```python
from build123d import *

# Parameters (mm, degrees)
SKETCH1_W             = 70
SKETCH1_H             = 5
BOSS_EXTRUDE1_DEPTH   = 36
SKETCH1_W_2           = 15
BOSS_EXTRUDE1_2_DEPTH = 36
SKETCH2_W             = 6
SKETCH2_H             = 70
BOSS_EXTRUDE2_DEPTH   = 70
M2_TAPPED_HOLE1_D     = 1.6
M2_TAPPED_HOLE1_DEPTH = 5
M2_TAPPED_HOLE1_TIP   = 0.480688495
M3_TAPPED_HOLE1_D     = 2.5
M2_5_TAPPED_HOLE1_D   = 2.05
SKETCH10_W            = 16.15
SKETCH10_H            = 7.752972879
CUT_EXTRUDE1_DEPTH    = 10


with BuildPart() as part:
    # Sketch1 → Boss-Extrude1 (new body)
    with BuildSketch(Plane.XY):
        with Locations((-4.38247012, 44.37250996)):
            Rectangle(SKETCH1_W, SKETCH1_H)
    extrude(amount=BOSS_EXTRUDE1_DEPTH)



with BuildPart() as body_2:
    # Sketch1 → Boss-Extrude1 2 (new body)
    with BuildSketch(Plane.XY):
        with Locations((23.11752988, -20.62749004)):
            Rectangle(SKETCH1_W_2, SKETCH1_H)
    extrude(amount=BOSS_EXTRUDE1_2_DEPTH)


with BuildPart() as part_1:
    add(part.part)

    add(body_2.part)  # Boss-Extrude2 merges body 2
    # Sketch2 → Boss-Extrude2 (add)
    with BuildSketch(Plane(origin=(30.61752988, 0, 0), x_dir=(0, 0, -1), z_dir=(1, 0, 0))):
        with Locations((-39, 11.87250996)):
            Rectangle(SKETCH2_W, SKETCH2_H)
    extrude(amount=-BOSS_EXTRUDE2_DEPTH)

    # M2 Tapped Hole1
    with Locations(Plane(origin=(23.61752988, 44.37250996, 0), x_dir=(-1, 0, 0), z_dir=(0, 0, -1))):
        with Locations((0, 0), (56, 0), (0, -65)):
            Hole(M2_TAPPED_HOLE1_D / 2, depth=M2_TAPPED_HOLE1_DEPTH)
            with Locations((0, 0, -(M2_TAPPED_HOLE1_DEPTH + M2_TAPPED_HOLE1_TIP / 2))):  # 118° drill point
                Cone(0, M2_TAPPED_HOLE1_D / 2, M2_TAPPED_HOLE1_TIP, mode=Mode.SUBTRACT)

    # M3 Tapped Hole1 (through all)
    with Locations(Plane(origin=(15.767468025, 11.87250996, 42), x_dir=(0, 1, 0), z_dir=(0, 0, 1))):
        with Locations((0, 0), (-10, -10), (10, -10)):
            Hole(M3_TAPPED_HOLE1_D / 2)

    # M2.5 Tapped Hole1 (through all)
    with Locations(Plane(origin=(-31.46932371, 28.191052792, 42), x_dir=(0, 1, 0), z_dir=(0, 0, 1))):
        with Locations((0, 0), (0, -20.15), (-33.4, -20.15), (-33.4, 0)):
            Hole(M2_5_TAPPED_HOLE1_D / 2)

    # Sketch10 → Cut-Extrude1 (cut)
    with BuildSketch(Plane.XY.offset(42)):
        with Locations((-21.39432371, 27.591449479)):
            Rectangle(SKETCH10_W, SKETCH10_H)
    extrude(amount=-CUT_EXTRUDE1_DEPTH, mode=Mode.SUBTRACT)


solid = part_1.part
```
Input: part model. Units: mm. Frame: model coordinates. A direction names the side the tool comes from. Round coordinates to 2 decimals unless told otherwise and drop trailing zeros. Write each loop counter-clockwise with the first axis right and the second up, starting at its lowest first coordinate (ties: lowest second). Pieces come first, ordered by that corner, then holes. Notation, with made-up numbers: (78.5, 15.25) -> (112.5, 15.25) arc R29 ccw to (112.5, 42.25) -> close; hole circle Ø6 at (29.5, 62). An arc over 180 degrees is marked (long way). Answer as CSV lines item,"result".
1. Contact query for flat-ended pins moving along their axis: P1, Ø4, axis at x = -1, z = 15, coming from the -Y side; P2, Ø1.2, axis at x = -11.32, y = 28.19, coming from the +Z side; P3, Ø5.5, axis at y = -21.5, z = 10.5, coming from the -X side; P4, Ø2.5, axis at x = -11.32, y = -5.21, coming from the -Z side. Output: stop coordinate, or through.
Geometry says:
P1,"stops at y = 41.87"
P2,"passes through"
P3,"stops at x = 15.62"
P4,"stops at z = 36"
2. Section C-C (z = 9.5). Return the cut outline in (x, y), plus the area to 3 significant figures.
Geometry says:
outline,"(-39.38, 41.87) -> (30.62, 41.87) -> (30.62, 46.87) -> (-39.38, 46.87) -> close; (15.62, -23.13) -> (30.62, -23.13) -> (30.62, -18.13) -> (15.62, -18.13) -> close"
area,"425 mm^2"
3. Reachability of faces 1 (the flat face through (-5, 41.873, 18)), 2 (the flat face through (-5, 44, 0)), 3 (the flat face through (-29.469, 28, 39)), 4 (the flat face through (15.618, -21, 18)) from +Z, -Z, +X, -X, +Y, -Y: full face, straight path, thin tool, end or side. Return the list, or none.
Geometry says:
face 1,"-Z, +X, -X"
face 2,"-Z, +X, -X, +Y, -Y"
face 3,"+Z, -Z"
face 4,"-Z, -X, -Y"
4. Section A-A (y = 25). Return the cut outline in (x, z), plus the area to 3 significant figures.
Geometry says:
outline,"(-39.38, 36) -> (-29.47, 36) -> (-29.47, 42) -> (-39.38, 42) -> close; (-13.32, 36) -> (30.62, 36) -> (30.62, 42) -> (-13.32, 42) -> close"
area,"323 mm^2"
5. Mould query, pull axis X, two halves, no side actions, for faces 5 (the flat face through (30.618, 9, 37)), 6 (the cylindrical face through (-30.56, 27.72, 38.96)), 7 (the flat face through (23, -18.127, 18)). Classes: +X half, -X half, draft (parallel to the pull), parting line (faces both ways), or undercut.
Geometry says:
face 5,"+X half"
face 6,"undercut"
face 7,"draft"
6. Ray query, L1, parallel to Y at x = 16, z = 30; L2, parallel to Y at x = -25.5, z = 15; L3, parallel to Z at x = -22.5, y = -13. Return the intervals inside material, ascending. Write a range as [from, to].
Geometry says:
L1,"y = [-23.13, -18.13], [41.87, 46.87]"
L2,"y = [41.87, 46.87]"
L3,"z = [36, 42]"
7. Section B-B (x = -23). Return the cut outline in (y, z).
Geometry says:
outline,"(-23.13, 36) -> (23.71, 36) -> (23.71, 42) -> (-23.13, 42) -> close; (31.47, 36) -> (41.87, 36) -> (41.87, 0) -> (46.87, 0) -> (46.87, 42) -> (31.47, 42) -> close"
8. Section D-D (z = 38). Give the number of separate pieces and of enclosed holes in the cut face, plus the area to 3 significant figures.
Geometry says:
separate pieces,"1"
enclosed holes,"8"
area,"4,750 mm^2"
